Design review of the part built by this model. Coordinates are the model's own, in mm. A direction names the side the tool comes from. Give positions to 0.01 mm unless a question says otherwise; leave off trailing zeros. Write each loop counter-clockwise with the first axis right and the second up, starting at its lowest first coordinate (ties: lowest second). Pieces come first, ordered by that corner, then holes.
```python
from build123d import *

# Parameters (mm, degrees)
BOSS_EXTRUDE1_DEPTH = 17.6
CUT_EXTRUDE1_DEPTH  = 15.6
SKETCH3_R           = 3
SKETCH3_R_2         = 2.5
BOSS_EXTRUDE2_DEPTH = 14.05
SKETCH4_W           = 6
SKETCH4_H           = 2.3
CUT_EXTRUDE2_DEPTH  = 14.05
SKETCH5_R           = 1.1
CUT_EXTRUDE3_DEPTH  = 12
SKETCH6_R           = 3.75
SKETCH6_R_2         = 2.6
SKETCH6_R_3         = 1.5
SKETCH6_R_4         = 1.25
SKETCH6_W           = 31.2
SKETCH6_H           = 41.4
CUT_EXTRUDE4_DEPTH  = 2
SKETCH7_W           = 3.5
SKETCH7_H           = 13.01
CUT_EXTRUDE5_DEPTH  = 14.35
SKETCH8_W           = 3.5
SKETCH8_H           = 21.74
CUT_EXTRUDE6_DEPTH  = 10
SKETCH9_W           = 3.5
SKETCH9_H           = 12.6
CUT_EXTRUDE7_DEPTH  = 6.135
SKETCH10_W          = 2.5
SKETCH10_H          = 3.5
CUT_EXTRUDE8_DEPTH  = 3.5


with BuildPart() as part:
    # Sketch1 → Boss-Extrude1 (new body)
    with BuildSketch(Plane.XY):
        with BuildLine():
            Line((-30, -36), (30, -36))
            ThreePointArc((30, -36), (34.242640687, -34.242640687), (36, -30))
            Line((36, -30), (36, 30))
            ThreePointArc((36, 30), (34.242640687, 34.242640687), (30, 36))
            Line((30, 36), (-30, 36))
            ThreePointArc((-30, 36), (-34.242640687, 34.242640687), (-36, 30))
            Line((-36, 30), (-36, -30))
            ThreePointArc((-36, -30), (-34.242640687, -34.242640687), (-30, -36))
        make_face()
    extrude(amount=BOSS_EXTRUDE1_DEPTH)

    # Sketch2 → Cut-Extrude1 (cut)
    with BuildSketch(Plane.XY):
        with BuildLine():
            Line((-30, -34), (30, -34))
            ThreePointArc((30, -34), (32.828427125, -32.828427125), (34, -30))
            Line((34, -30), (34, 30))
            ThreePointArc((34, 30), (32.828427125, 32.828427125), (30, 34))
            Line((30, 34), (-30, 34))
            ThreePointArc((-30, 34), (-32.828427125, 32.828427125), (-34, 30))
            Line((-34, 30), (-34, -30))
            ThreePointArc((-34, -30), (-32.828427125, -32.828427125), (-30, -34))
        make_face()
    extrude(amount=CUT_EXTRUDE1_DEPTH, mode=Mode.SUBTRACT)

    # Sketch3 → Boss-Extrude2 (add)
    with BuildSketch(Plane.XY.offset(1.55)):
        with Locations(Location((-30, 30, 0), (0, 0, 180))):
            Circle(SKETCH3_R)
        with Locations(Location((30, 30, 0), (0, 0, 180))):
            Circle(SKETCH3_R_2)
        with Locations(Location((-30, -30, 0), (0, 0, 180))):
            Circle(SKETCH3_R)
        with Locations(Location((30, -30, 0), (0, 0, 180))):
            Circle(SKETCH3_R)
    extrude(amount=BOSS_EXTRUDE2_DEPTH)

    # Sketch4 → Cut-Extrude2 (cut)
    with BuildSketch(Plane.XY.offset(1.55)):
        with Locations((30, 27.15)):
            Rectangle(SKETCH4_W, SKETCH4_H)
    extrude(amount=CUT_EXTRUDE2_DEPTH, mode=Mode.SUBTRACT)

    # Sketch5 → Cut-Extrude3 (cut)
    with BuildSketch(Plane.XY.offset(1.55)):
        with Locations((-30, 30)):
            Circle(SKETCH5_R)
        with Locations((30, 30)):
            Circle(SKETCH5_R)
        with Locations((-30, -30)):
            Circle(SKETCH5_R)
        with Locations((30, -30)):
            Circle(SKETCH5_R)
    extrude(amount=CUT_EXTRUDE3_DEPTH, mode=Mode.SUBTRACT)

    # Sketch6 → Cut-Extrude4 (cut)
    with BuildSketch(Plane.XY.offset(15.6)):
        with Locations((-25, 18)):
            Circle(SKETCH6_R)
        with Locations((-25, 3)):
            Circle(SKETCH6_R_2)
        with Locations((-25, -7)):
            Circle(SKETCH6_R_2)
        with Locations((0, 30.5)):
            Circle(SKETCH6_R_3)
        with Locations((-28.5, -12.1)):
            Circle(SKETCH6_R_4)
        with Locations((29.5, -11)):
            Circle(SKETCH6_R_4)
        Rectangle(SKETCH6_W, SKETCH6_H)
        with BuildLine():
            Line((30.5, 24.5), (30.5, 9.5))
            ThreePointArc((30.5, 9.5), (28.25, 7.25), (26, 9.5))
            Line((26, 9.5), (26, 24.5))
            ThreePointArc((26, 24.5), (28.25, 26.75), (30.5, 24.5))
        make_face()
        with BuildLine():
            Line((-11.1, -23.5), (-11.1, -31.5))
            ThreePointArc((-11.1, -31.5), (-12, -32.4), (-12.9, -31.5))
            Line((-12.9, -31.5), (-12.9, -23.5))
            ThreePointArc((-12.9, -23.5), (-12, -22.6), (-11.1, -23.5))
        make_face()
        with BuildLine():
            Line((-7.1, -23.5), (-7.1, -31.5))
            ThreePointArc((-7.1, -31.5), (-8, -32.4), (-8.9, -31.5))
            Line((-8.9, -31.5), (-8.9, -23.5))
            ThreePointArc((-8.9, -23.5), (-8, -22.6), (-7.1, -23.5))
        make_face()
        with BuildLine():
            Line((-3.1, -23.5), (-3.1, -31.5))
            ThreePointArc((-3.1, -31.5), (-4, -32.4), (-4.9, -31.5))
            Line((-4.9, -31.5), (-4.9, -23.5))
            ThreePointArc((-4.9, -23.5), (-4, -22.6), (-3.1, -23.5))
        make_face()
        with BuildLine():
            Line((0.9, -23.5), (0.9, -31.5))
            ThreePointArc((0.9, -31.5), (0, -32.4), (-0.9, -31.5))
            Line((-0.9, -31.5), (-0.9, -23.5))
            ThreePointArc((-0.9, -23.5), (0, -22.6), (0.9, -23.5))
        make_face()
        with BuildLine():
            Line((4.9, -23.5), (4.9, -31.5))
            ThreePointArc((4.9, -31.5), (4, -32.4), (3.1, -31.5))
            Line((3.1, -31.5), (3.1, -23.5))
            ThreePointArc((3.1, -23.5), (4, -22.6), (4.9, -23.5))
        make_face()
        with BuildLine():
            Line((8.9, -23.5), (8.9, -31.5))
            ThreePointArc((8.9, -31.5), (8, -32.4), (7.1, -31.5))
            Line((7.1, -31.5), (7.1, -23.5))
            ThreePointArc((7.1, -23.5), (8, -22.6), (8.9, -23.5))
        make_face()
        with BuildLine():
            Line((12.9, -23.5), (12.9, -31.5))
            ThreePointArc((12.9, -31.5), (12, -32.4), (11.1, -31.5))
            Line((11.1, -31.5), (11.1, -23.5))
            ThreePointArc((11.1, -23.5), (12, -22.6), (12.9, -23.5))
        make_face()
    extrude(amount=CUT_EXTRUDE4_DEPTH, mode=Mode.SUBTRACT)

    # Sketch7 → Cut-Extrude5 (cut)
    with BuildSketch(Plane.XY):
        with Locations((35.25, -1.445)):
            Rectangle(SKETCH7_W, SKETCH7_H)
        with Locations((35.25, -20.495)):
            Rectangle(SKETCH7_W, SKETCH7_H)
    extrude(amount=CUT_EXTRUDE5_DEPTH, mode=Mode.SUBTRACT)

    # Sketch8 → Cut-Extrude6 (cut)
    with BuildSketch(Plane.XY):
        with Locations((35.25, 17.53)):
            Rectangle(SKETCH8_W, SKETCH8_H)
    extrude(amount=CUT_EXTRUDE6_DEPTH, mode=Mode.SUBTRACT)

    # Sketch9 → Cut-Extrude7 (cut)
    with BuildSketch(Plane.XY):
        with Locations((-35.25, -19)):
            Rectangle(SKETCH9_W, SKETCH9_H)
    extrude(amount=CUT_EXTRUDE7_DEPTH, mode=Mode.SUBTRACT)

    # Sketch10 → Cut-Extrude8 (cut)
    with BuildSketch(Plane.XY):
        with Locations((-11, 35.25)):
            Rectangle(SKETCH10_W, SKETCH10_H)
        with Locations((11, 35.25)):
            Rectangle(SKETCH10_W, SKETCH10_H)
    extrude(amount=CUT_EXTRUDE8_DEPTH, mode=Mode.SUBTRACT)


solid = part.part
```
(1) Consider section D-D, the plane x = -24. Give the boundary of the cut face in (y, z).
Resolved:
outline: (-36, 0) - (-34, 0) - (-34, 15.6) - (-9.4, 15.6) - (-9.4, 17.6) - (-36, 17.6) - close; (-4.6, 15.6) - (0.6, 15.6) - (0.6, 17.6) - (-4.6, 17.6) - close; (5.4, 15.6) - (14.39, 15.6) - (14.39, 17.6) - (5.4, 17.6) - close; (21.61, 15.6) - (34, 15.6) - (34, 0) - (36, 0) - (36, 17.6) - (21.61, 17.6) - close
(2) Consider section C-C, the plane y = 12.5. Give the boundary of the cut face in (x, z), then the cut area to 3 significant figures.
Resolved:
outline: (-36, 0) - (-34, 0) - (-34, 15.6) - (-15.6, 15.6) - (-15.6, 17.6) - (-36, 17.6) - close; (15.6, 15.6) - (26, 15.6) - (26, 17.6) - (15.6, 17.6) - close; (30.5, 15.6) - (34, 15.6) - (34, 10) - (36, 10) - (36, 17.6) - (30.5, 17.6) - close
area: 115 mm2
(3) Mouldability with a two-part tool opening along X and no side actions: class faces 4 (the face through (30, 28.3, 8)), 5 (the face through (35, -1, 14.35)), 6 (the face through (30, -28.7, 1.55)), 7 (the face through (-34.196, 34.289, 8.677)) as pulls with the +X half, pulls with the -X half, needs draft (parallel to the pull), parting line crosses it, or undercut.
Resolved:
face 4: undercut
face 5: needs draft
face 6: undercut
face 7: pulls with the -X half
(4) Clearance check with flat-ended pins moving along their axes: P1, Ø1.6, axis at x = 34.5, y = -2, coming from the -Z side; P2, Ø0.6, axis at x = -35.5, z = 4, coming from the +Y side; P3, Ø1.3, axis at x = 29.5, y = 29.5, coming from the -Z side; P4, Ø4.5, axis at x = -25, y = 18, coming from the -Z side. State where each tip first meets the part, or that it passes through.
Resolved:
P1: stops at z = 14.35
P2: stops at y = 32.99
P3: stops at z = 1.55
P4: passes through
(5) Consider section A-A, the plane y = -16. Give the boundary of the cut face in (x, z) (3 decimals).
Resolved:
outline: (-36, 6.135) - (-34, 6.135) - (-34, 15.6) - (-15.6, 15.6) - (-15.6, 17.6) - (-36, 17.6) - close; (15.6, 15.6) - (34, 15.6) - (34, 14.35) - (36, 14.35) - (36, 17.6) - (15.6, 17.6) - close
(6) To check wall thickness, follow L1, parallel to Y at x = -25, z = 16.3; L2, parallel to Y at x = 15.5, z = 12.75. State the ranges of each line that lie inside material, in increasing order.
Resolved:
L1: y = -36 to -9.6, -4.4 to 0.4, 5.6 to 14.25, 21.75 to 36
L2: y = -36 to -34, 34 to 36
(7) Consider section B-B, the plane x = 4. Give the boundary of the cut face in (y, z), then the cut area to 3 significant figures.
Resolved:
outline: (-36, 0) - (-34, 0) - (-34, 15.6) - (-32.4, 15.6) - (-32.4, 17.6) - (-36, 17.6) - close; (-22.6, 15.6) - (-20.7, 15.6) - (-20.7, 17.6) - (-22.6, 17.6) - close; (20.7, 15.6) - (34, 15.6) - (34, 0) - (36, 0) - (36, 17.6) - (20.7, 17.6) - close
area: 104 mm2
(8) Tool access review of faces 1 (the face through (-34, 0, 8)), 2 (the face through (4, -22.6, 16.6)), 3 (the face through (-11, 35, 3.5)): name each direction out of +Z, -Z, +X, -X, +Y, -Y from which nothing blocks a thin tool from reaching the whole face with its end or side.
Resolved:
face 1: -Z
face 2: +Z, -Z
face 3: -Z, +Y
